```python
from build123d import *

# Parameters (mm, degrees)
CUT_EXTRUDE1_DEPTH = 1
CHAMFER1_SIZE      = 0.125


with BuildPart() as part:
    # Sketch1 → Revolve1 (revolve)
    with BuildSketch(Plane(origin=(0, 0, 0), x_dir=(1, 0, 0), z_dir=(0, 1, 0))):
        Polygon((0, 0), (0, 7), (1.25, 7), (1.25, 2.5), (1.5, 2.5), (1.5, 1), (2.25, 1), (2.25, 0), align=None)
    revolve(axis=Axis((0, 0, 0), (0, 0, 1)))

    # Sketch2 → Cut-Extrude1 (cut)
    with BuildSketch(Plane.XY):
        Polygon((1.154700538, 0), (0.577350269, 1), (-0.577350269, 1), (-1.154700538, 0), (-0.577350269, -1), (0.577350269, -1), align=None)
    extrude(amount=-CUT_EXTRUDE1_DEPTH, mode=Mode.SUBTRACT)

    # Chamfer1
    chamfer1_edges = [part.edges().sort_by_distance(p)[0] for p in [
        (-2.25, 0, 0),
        (-1.5, 0, -2.5),
        (-1.25, 0, -7),
    ]]
    chamfer(chamfer1_edges, length=CHAMFER1_SIZE)


solid = part.part
```
Work out the finished part from the listing and answer in its coordinate system (mm). A direction names the side the tool comes from. Round coordinates to 2 decimals unless told otherwise and drop trailing zeros. Loops run counter-clockwise (first coordinate to the right, second up) from the corner with the lowest first, then second, coordinate; pieces in that order, holes last. Notation, with made-up numbers: M 14,89 L 64,89 A32 ccw 64,122 Z; hole C 56,89.25 d5. An arc over 180 degrees is marked long. One line per question, with ' | ' between items.
Q1. Consider line 1 along Y through (x, z) = (-0.55, -5.25); line 2 along Z through (x, y) = (1.15, -1.35); line 3 along Y through (x, z) = (0, -4.25). Determine where each line is inside the solid, lowest interval first. Write a range as from..to.
Conclusion:
line 1: y = -1.12..1.12 | line 2: z = -1..0 | line 3: y = -1.25..1.25
Q2. Find section A-A, the plane z = -0.5. Give the vertices of the cut face in (x, y), then the cut area to 3 significant figures.
Conclusion:
outline: C 0,0 d4.5; hole M -1.15,0 L -0.58,-1 L 0.58,-1 L 1.15,0 L 0.58,1 L -0.58,1 Z | area: 12.4 mm2
Q3. The mould has two halves that part along X. Classify faces 1 (the flat face through (0, -1, -0.5)), 2 (the cylindrical face through (-1.5, 0.07, -1.68)), 3 (the flat face through (2, 0, -1)): +X half, -X half, draft (parallel to the pull), parting line (faces both ways), or undercut.
Conclusion:
face 1: undercut | face 2: parting line | face 3: draft
Q4. Each of these flat-tipped pins is pushed along its axis until it touches: pin 1 Ø1.6 at (x, y) = (0, 0) entering from +Z; pin 2 Ø0.5 at (x, z) = (0.5, -0.5) entering from -Y. Where does it stop, or does it pass through?
Conclusion:
pin 1: stops at z = -1 | pin 2: stops at y = -2.24
Q5. Find section C-C, the plane z = -1.5. Give the vertices of the cut face in (x, y).
Conclusion:
outline: C 0,0 d3
Q6. Find section B-B, the plane x = 0. Give the vertices of the cut face in (y, z) (3 decimals).
Conclusion:
outline: M -2.25,-1 L -1.5,-1 L -1.5,-2.375 L -1.375,-2.5 L -1.25,-2.5 L -1.25,-6.875 L -1.125,-7 L 1.125,-7 L 1.25,-6.875 L 1.25,-2.5 L 1.375,-2.5 L 1.5,-2.375 L 1.5,-1 L 2.25,-1 L 2.25,-0.125 L 2.125,0 L 1,0 L 1,-1 L -1,-1 L -1,0 L -2.125,0 L -2.25,-0.125 Z
Q7. A tool of negligible diameter and unlimited length cuts with its end or side. For faces 4 (the flat face through (1, 1, 0)), 5 (the flat face through (0, 0, -1)), 6 (the cylindrical face through (-0.27, -1.22, -4.66)), from which of +Z, -Z, +X, -X, +Y, -Y can it reach the whole face along a straight path? Write none if from no direction.
Conclusion:
face 4: +Z, +X, -X, +Y, -Y | face 5: +Z | face 6: -Z
Q8. Find section D-D, the plane z = -4. Give the vertices of the cut face in (x, y).
Conclusion:
outline: C 0,0 d2.5
